Input: part model. Units: mm. Frame: model coordinates. Face numbers are marked on the shaded views. A direction names the side the tool comes from. Coordinates: 2 decimals unless noted, no trailing zeros. Loops run counter-clockwise (first coordinate to the right, second up) from the corner with the lowest first, then second, coordinate; pieces in that order, holes last. Notation, with made-up numbers: (84, 87.5) - (121, 87.5) arc R17 cw to (121, 99.5) - close; hole circle Ø11 at (67.25, 53.5). An arc over 180 degrees is marked (long way). Use a Markdown table: item, result. Add a question column.
1. Draft query along Z for the marked faces 1, 2 and 3. Return one class per face: released by +Z, released by -Z, zero draft, split by the parting line, or undercut.
2. Access query for the marked faces 4, 5, 6 and 7. Directions: +Z, -Z, +X, -X, +Y, -Y. A direction counts if a zero-diameter tool reaches every point of the face in a straight line with its end or side. Return the directions, or none.
3. Section query B-B on z = -4. Return the cut outline in (x, y), then the cut area to 3 significant figures.
4. Section query A-A on y = 11.5. Return the cut outline in (x, z), then the cut area to 3 significant figures.
5. Section query C-C on y = -1. Return the cut outline in (x, z).
6. Ray query, L1, parallel to Z at x = 2.45, y = 11.5; L2, parallel to Y at x = 3.65, z = -4; L3, parallel to Y at x = 2.6, z = 0. Return the intervals inside material, ascending. Write a range as [from, to].
7. Contact query for flat-ended pins moving along their axis: P1, Ø2.5, axis at x = 1.5, z = 6.5, coming from the +Y side; P2, Ø2, axis at y = 17, z = -4, coming from the -X side; P3, Ø1.5, axis at x = 2, y = 10, coming from the +Z side; P4, Ø3, axis at y = 26, z = 1, coming from the -X side. Output: stop coordinate, or through.
8. Section query D-D on x = 0.65. State how many separate pieces and enclosed holes the cut face has, then the cut area to 3 significant figures.
```python
from build123d import *

# Parameters (mm, degrees)
SKETCH1_R                   = 2.05
SKETCH1_R_2                 = 1.5
BOSS_EXTRUDE1_DEPTH         = 5
FILLET1_START               = -1
FILLET1_DEPTH               = 7
FILLET1_2_DEPTH             = 5
TAP_DRILL_FOR_M2X0_4_TAP1_D = 1.6
SKETCH4_W                   = 9
SKETCH4_H                   = 9
CUT_EXTRUDE1_DEPTH          = 2
SKETCH5_R                   = 5
CUT_EXTRUDE2_DEPTH          = 3.5


with BuildPart() as part:
    # Sketch1 → Boss-Extrude1 (new body)
    with BuildSketch(Plane(origin=(0, 0, 0), x_dir=(0, 0, -1), z_dir=(1, 0, 0))):
        with BuildLine():
            Line((6, 0), (6, 28))
            ThreePointArc((6, 28), (4.242640687, 32.242640687), (0, 34))
            Line((0, 34), (-9.875644347, 34))
            ThreePointArc((-9.875644347, 34), (-14.875644347, 35.339745962), (-18.535898385, 39))
            Line((-18.535898385, 39), (-21.084936491, 43.415063509))
            Line((-21.084936491, 43.415063509), (-25.415063509, 40.915063509))
            Line((-25.415063509, 40.915063509), (-17.260063509, 26.790189174))
            ThreePointArc((-17.260063509, 26.790189174), (-16.528012702, 26.058138366), (-15.528012702, 25.790189174))
            Line((-15.528012702, 25.790189174), (-13, 25.790189174))
            ThreePointArc((-13, 25.790189174), (-5.928932188, 22.861256986), (-3, 15.790189174))
            Line((-3, 15.790189174), (-3, 3))
            Line((-3, 3), (-5, 3))
            Line((-5, 3), (-5, -3.31662479))
            ThreePointArc((-5, -3.31662479), (1.732050808, -5.744562647), (6, 0))
        make_face()
        Circle(SKETCH1_R, mode=Mode.SUBTRACT)
        with Locations((-22, 40)):
            Circle(SKETCH1_R_2, mode=Mode.SUBTRACT)
        with Locations((-17, 31.339745962)):
            Circle(SKETCH1_R_2, mode=Mode.SUBTRACT)
        with Locations((-1, 11.5)):
            Circle(SKETCH1_R_2, mode=Mode.SUBTRACT)
        with Locations((4, 11.5)):
            Circle(SKETCH1_R_2, mode=Mode.SUBTRACT)
        with Locations((4, 7.5)):
            Circle(SKETCH1_R_2, mode=Mode.SUBTRACT)
    extrude(amount=BOSS_EXTRUDE1_DEPTH)

    # Fillet1: read off the stored shape, not the designer's step
    # Fillet1 outline → Fillet1 (cut)
    with BuildSketch(Plane.YZ.offset(FILLET1_START)):
        with BuildLine():
            ThreePointArc((2, 5), (2.707106781, 4.707106781), (3, 4))
            Line((3, 4), (3, 5))
            Line((3, 5), (2, 5))
        make_face()
    extrude(amount=FILLET1_DEPTH, mode=Mode.SUBTRACT)

    # Fillet1 2 outline → Fillet1 2 (add)
    with BuildSketch(Plane.YZ):
        with BuildLine():
            ThreePointArc((4, 3), (3.292893219, 3.292893219), (3, 4))
            Line((3, 4), (3, 3))
            Line((3, 3), (4, 3))
        make_face()
    extrude(amount=FILLET1_2_DEPTH)

    # Tap Drill for M2x0.4 Tap1 (through all)
    with Locations(Plane(origin=(5, 0, 0), x_dir=(0, 0, -1), z_dir=(1, 0, 0))):
        with Locations((-1.2, 17), (4, 17)):
            Hole(TAP_DRILL_FOR_M2X0_4_TAP1_D / 2)

    # Sketch4 → Cut-Extrude1 (cut)
    with BuildSketch(Plane.ZY.offset(-5)):
        with Locations((-1.5, 9.5)):
            Rectangle(SKETCH4_W, SKETCH4_H)
    extrude(amount=CUT_EXTRUDE1_DEPTH, mode=Mode.SUBTRACT)

    # Sketch5 → Cut-Extrude2 (cut)
    with BuildSketch(Plane(origin=(0, 0, 0), x_dir=(0, 0, -1), z_dir=(1, 0, 0))):
        with Locations((0, 28)):
            Circle(SKETCH5_R)
    extrude(amount=CUT_EXTRUDE2_DEPTH, mode=Mode.SUBTRACT)


solid = part.part
```
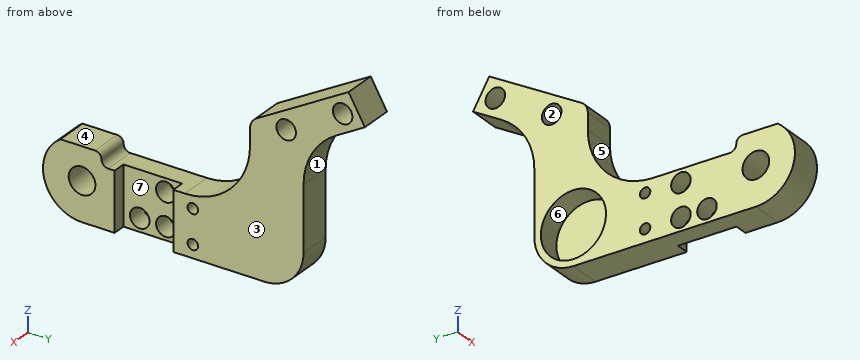
Resolved:
| question | item | result |
|---|---|---|
| 1 | face 1 | released by -Z |
| 1 | face 2 | undercut |
| 1 | face 3 | zero draft |
| 2 | face 4 | +Z, +X, -X, -Y |
| 2 | face 5 | +Z, +X, -X |
| 2 | face 6 | -X |
| 2 | face 7 | +Z, -Z, +X |
| 3 | outline | (0, -4.47) - (5, -4.47) - (5, 5) - (3, 5) - (3, 6) - (0, 6) - close; (0, 9) - (3, 9) - (3, 10) - (0, 10) - close; (0, 13) - (3, 13) - (3, 14) - (5, 14) - (5, 16.2) - (0, 16.2) - close; (0, 17.8) - (5, 17.8) - (5, 32.47) - (0, 32.47) - (0, 31) - (3.5, 31) - (3.5, 25) - (0, 25) - close |
| 3 | area | 120 mm² |
| 4 | outline | (0, -6) - (3, -6) - (3, -5.5) - (0, -5.5) - close; (0, -2.5) - (3, -2.5) - (3, -0.5) - (0, -0.5) - close; (0, 2.5) - (3, 2.5) - (3, 3) - (0, 3) - close |
| 4 | area | 9.00 mm² |
| 5 | outline | (0, -5.92) - (5, -5.92) - (5, -1.79) - (0, -1.79) - close; (0, 1.79) - (5, 1.79) - (5, 5) - (0, 5) - close |
| 6 | L1 | [-6, -5.5], [-2.5, -0.5], [2.5, 3] |
| 6 | L2 | [-4.47, 5], [14, 16.2], [17.8, 32.47] |
| 6 | L3 | [-6, -2.05], [2.05, 10.38], [12.62, 23], [33, 34] |
| 7 | P1 | y = 34 |
| 7 | P2 | x = 0 |
| 7 | P3 | z = 3 |
| 7 | P4 | x = 3.5 |
| 8 | separate pieces | 1 |
| 8 | enclosed holes | 9 |
| 8 | area | 433 mm² |
